from build123d import *

# Parameters (mm, degrees)
SKETCH2_W                    = 75
SKETCH2_H                    = 80
BASE_FLANGE1_DEPTH           = 0.6
CUT_EXTRUDE1_REACH           = 111.66
SKETCH10_R                   = 2.5
EDGE_FLANGE1_STRIP_W         = 3.8732
EDGE_FLANGE1_STRIP_H         = 0.6
EDGE_FLANGE1_STRIP_CUT_DEPTH = 75
EDGE_FLANGE1_DEPTH           = 75


# Sheet-metal steps are written as plain solids
with BuildPart() as part:
    # Sketch2 → Base-Flange1 (new body)
    with BuildSketch(Plane.XY):
        with Locations((37.5, 40)):
            Rectangle(SKETCH2_W, SKETCH2_H)
    extrude(amount=-BASE_FLANGE1_DEPTH)

    # Sketch10 → Cut-Extrude1 (cut, up to next)
    with BuildSketch(Plane(origin=(0, 0, -0.6), x_dir=(-1, 0, 0), z_dir=(0, 0, -1)), mode=Mode.PRIVATE) as cut_extrude1_sk1:
        with Locations((-22.5, 10)):
            Circle(SKETCH10_R)
    cut_extrude1_tool1 = extrude(cut_extrude1_sk1.sketch, amount=-CUT_EXTRUDE1_REACH, mode=Mode.PRIVATE) & part.part
    # Sketch10 → Cut-Extrude1 (cut, up to next)
    with BuildSketch(Plane(origin=(0, 0, -0.6), x_dir=(-1, 0, 0), z_dir=(0, 0, -1)), mode=Mode.PRIVATE) as cut_extrude1_sk2:
        with Locations((-52.5, 70)):
            Circle(SKETCH10_R)
    cut_extrude1_tool2 = extrude(cut_extrude1_sk2.sketch, amount=-CUT_EXTRUDE1_REACH, mode=Mode.PRIVATE) & part.part
    # Sketch10 → Cut-Extrude1 (cut, up to next)
    with BuildSketch(Plane(origin=(0, 0, -0.6), x_dir=(-1, 0, 0), z_dir=(0, 0, -1)), mode=Mode.PRIVATE) as cut_extrude1_sk3:
        with Locations((-52.5, 10)):
            Circle(SKETCH10_R)
    cut_extrude1_tool3 = extrude(cut_extrude1_sk3.sketch, amount=-CUT_EXTRUDE1_REACH, mode=Mode.PRIVATE) & part.part
    # Sketch10 → Cut-Extrude1 (cut, up to next)
    with BuildSketch(Plane(origin=(0, 0, -0.6), x_dir=(-1, 0, 0), z_dir=(0, 0, -1)), mode=Mode.PRIVATE) as cut_extrude1_sk4:
        with Locations((-22.5, 70)):
            Circle(SKETCH10_R)
    cut_extrude1_tool4 = extrude(cut_extrude1_sk4.sketch, amount=-CUT_EXTRUDE1_REACH, mode=Mode.PRIVATE) & part.part
    add(cut_extrude1_tool1.solids().sort_by_distance((22.5, 10, -0.6))[0], mode=Mode.SUBTRACT)
    add(cut_extrude1_tool2.solids().sort_by_distance((52.5, 70, -0.6))[0], mode=Mode.SUBTRACT)
    add(cut_extrude1_tool3.solids().sort_by_distance((52.5, 10, -0.6))[0], mode=Mode.SUBTRACT)
    add(cut_extrude1_tool4.solids().sort_by_distance((22.5, 70, -0.6))[0], mode=Mode.SUBTRACT)

    # Edge-Flange1 strip (across the edge) → Edge-Flange1 strip cut (cut)
    with BuildSketch(Plane.YZ):
        with Locations((-0.6, -0.3)):
            Rectangle(EDGE_FLANGE1_STRIP_W, EDGE_FLANGE1_STRIP_H)
    extrude(amount=EDGE_FLANGE1_STRIP_CUT_DEPTH, mode=Mode.SUBTRACT)

    # Edge-Flange1 section (across the edge) → Edge-Flange1 (add)
    with BuildSketch(Plane.YZ):
        with BuildLine():
            Line((0, 0.7366), (0, 73))
            Line((0, 73), (0.6, 73))
            Line((0.6, 73), (0.6, 0.7366))
            ThreePointArc((0.6, 0.7366), (0.815745145, 0.215745145), (1.3366, 0))
            Line((1.3366, 0), (1.3366, -0.6))
            ThreePointArc((1.3366, -0.6), (0.391481076, -0.208518924), (0, 0.7366))
        make_face()
    extrude(amount=EDGE_FLANGE1_DEPTH)


solid = part.part
Geometry: final body of the model. Coordinates: model frame, mm. A direction names the side the tool comes from. Round coordinates to 2 decimals unless told otherwise and drop trailing zeros. Order: outer loops, then holes, each group sorted by start corner. A loop starts at its lowest first (then second) coordinate and runs counter-clockwise, first axis right, second up. Notation, with made-up numbers: (-8.5, 70.25) - (45.5, 70.25) arc R30 ccw to (45.5, 107.25) - close; hole circle Ø1 at (-29, 43). An arc over 180 degrees is marked (long way). Write each question's results on one line, items separated by ' | '.
Item 1: Material intervals for line 1 along Y through (x, z) = (22.5, -0.3); line 2 along Y through (x, z) = (28, 59); line 3 along Y through (x, z) = (22.5, -0.25), sorted ascending. Write a range as [from, to].
Completed:
line 1: [0.49, 7.5], [12.5, 67.5], [72.5, 80] | line 2: [0, 0.6] | line 3: [0.43, 7.5], [12.5, 67.5], [72.5, 80]
Item 2: Section B-B, the plane x = 52.5. Return the cut outline in (y, z).
Completed:
outline: (0, 0.74) arc R1.34 ccw to (1.34, -0.6) - (7.5, -0.6) - (7.5, 0) - (1.34, 0) arc R0.74 cw to (0.6, 0.74) - (0.6, 73) - (0, 73) - close; (12.5, -0.6) - (67.5, -0.6) - (67.5, 0) - (12.5, 0) - close; (72.5, -0.6) - (80, -0.6) - (80, 0) - (72.5, 0) - close
Item 3: Section A-A, the plane y = 10. Return the cut outline in (x, z), and give its area (3 significant figures).
Completed:
outline: (0, -0.6) - (20, -0.6) - (20, 0) - (0, 0) - close; (25, -0.6) - (50, -0.6) - (50, 0) - (25, 0) - close; (55, -0.6) - (75, -0.6) - (75, 0) - (55, 0) - close | area: 39.0 mm^2
Item 4: First-contact query: pin 1 Ø21.5 at (x, z) = (32, 46) entering from +Y; pin 2 Ø1.5 at (x, y) = (58, 57.5) entering from +Z. Flat tips, straight axial feed; report the tip coordinate or a pass-through.
Completed:
pin 1: y = 0.6 | pin 2: z = 0
Item 5: Mould query, pull axis X, two halves, no side actions, for faces 1 (the flat face through (37, 0, 36)), 2 (the cylindrical face through (50.19, 69.04, -0.3)). Classes: pulls with the +X half, pulls with the -X half, needs draft (parallel to the pull), parting line crosses it, or undercut.
Completed:
face 1: needs draft | face 2: undercut
Item 6: Reachability of faces 3 (the flat face through (37, 0.6, 37)), 4 (the cylindrical face through (24.5, 68.5, -0.3)) from +Z, -Z, +X, -X, +Y, -Y: full face, straight path, thin tool, end or side. Return the list, or none.
Completed:
face 3: +Z, +X, -X, +Y | face 4: +Z, -Z
Item 7: Section D-D, the plane y = 35. Return the cut outline in (x, z), and give its area (3 significant figures).
Completed:
outline: (0, -0.6) - (75, -0.6) - (75, 0) - (0, 0) - close | area: 45.0 mm^2
Item 8: Section C-C, the plane x = 6. Return the cut outline in (y, z).
Completed:
outline: (0, 0.74) arc R1.34 ccw to (1.34, -0.6) - (80, -0.6) - (80, 0) - (1.34, 0) arc R0.74 cw to (0.6, 0.74) - (0.6, 73) - (0, 73) - close
